```python
from build123d import *

# Parameters (mm, degrees)
SKETCH1_W           = 20.32
SKETCH1_H           = 76.2
BOSS_EXTRUDE1_DEPTH = 22.86
SKETCH2_R           = 3.175
CUT_EXTRUDE1_DEPTH  = 92.1573409
SKETCH3_W           = 20.32
SKETCH3_H           = 45.72
BOSS_EXTRUDE2_DEPTH = 50.8
SKETCH4_R           = 17.999964
CUT_EXTRUDE2_DEPTH  = 17.78
SKETCH5_R           = 2.999994
CUT_EXTRUDE3_DEPTH  = 131.260155074


with BuildPart() as part:
    # Sketch1 → Boss-Extrude1 (new, symmetric)
    with BuildSketch(Plane.XY):
        with Locations((10.16, 38.1)):
            Rectangle(SKETCH1_W, SKETCH1_H)
    extrude(amount=BOSS_EXTRUDE1_DEPTH, both=True)

    # Sketch2 → Cut-Extrude1 (cut, through all)
    with BuildSketch(Plane.XY.offset(22.86)):
        with Locations((10.16, 12.7)):
            Circle(SKETCH2_R)
        with Locations((10.16, 38.1)):
            Circle(SKETCH2_R)
        with Locations((10.16, 63.5)):
            Circle(SKETCH2_R)
    extrude(amount=-CUT_EXTRUDE1_DEPTH, mode=Mode.SUBTRACT)

    # Sketch3 → Boss-Extrude2 (add)
    with BuildSketch(Plane(origin=(0, 76.2, 0), x_dir=(1, 0, 0), z_dir=(0, 1, 0))):
        with Locations((10.16, 0)):
            Rectangle(SKETCH3_W, SKETCH3_H)
    extrude(amount=BOSS_EXTRUDE2_DEPTH)

    # Sketch4 → Cut-Extrude2 (cut)
    with BuildSketch(Plane(origin=(20.32, 0, 0), x_dir=(0, 0, -1), z_dir=(1, 0, 0))):
        with Locations((0, 96.300036)):
            Circle(SKETCH4_R)
    extrude(amount=-CUT_EXTRUDE2_DEPTH, mode=Mode.SUBTRACT)

    # Sketch5 → Cut-Extrude3 (cut, through all)
    with BuildSketch(Plane(origin=(2.54, 0, 0), x_dir=(0, 0, -1), z_dir=(1, 0, 0))):
        with Locations((0, 96.300036)):
            Circle(SKETCH5_R)
    extrude(amount=-CUT_EXTRUDE3_DEPTH, mode=Mode.SUBTRACT)


solid = part.part
```
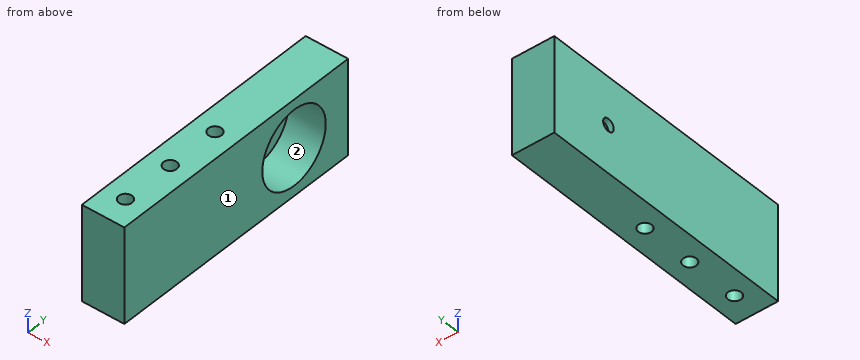
The listing builds one solid part. Answer for the finished solid, in the listing's coordinates (mm). Face numbers are marked on the shaded views. A direction names the side the tool comes from. Round coordinates to 2 decimals unless told otherwise and drop trailing zeros. Write each loop counter-clockwise with the first axis right and the second up, starting at its lowest first coordinate (ties: lowest second). Pieces come first, ordered by that corner, then holes. Notation, with made-up numbers: (14.25, 27) -> (70.25, 27) arc R14 cw to (70.25, 38) -> close; hole circle Ø10 at (79, 41). An arc over 180 degrees is marked (long way). Answer as a JSON object with one key per item and string values. Group by question number.
Q1. Section C-C (x = 10.16) is taken. Write down the section's boundary in (y, z) (3 decimals), plus the area to 3 significant figures.
Q2. Section D-D (z = -5) is taken. Write down the section's boundary in (x, y) (3 decimals), plus the area to 3 significant figures.
Q3. Section B-B (z = 0) is taken. Write down the section's boundary in (x, y) (3 decimals).
Q4. Each of these flat-tipped pins is pushed along its axis until it touches: pin 1 Ø12 at (y, z) = (71.5, -7) entering from -X; pin 2 Ø5.5 at (y, z) = (96.3, 0) entering from +X. Where does it stop, or does it pass through?
Q5. Straight lines are drawn through the part: line 1 along Y through (x, z) = (1.75, 0); line 2 along Y through (x, z) = (9.25, 0); line 3 along Y through (x, z) = (10.16, 7) (3 decimals). For each, find the intervals that lie inside material, in ascending order.
Q6. Section A-A (y = 63.5) is taken. Write down the section's boundary in (x, z) (3 decimals), plus the area to 3 significant figures.
Q7. Which of the six approach directions +Z, -Z, +X, -X, +Y, -Y give full straight-line access (tool end or side, diameter ignored) to the marked faces 1 and 2?
Check values:
{
 "1": {"outline": "(0, -22.86) -> (9.525, -22.86) -> (9.525, 22.86) -> (0, 22.86) -> close; (15.875, -22.86) -> (34.925, -22.86) -> (34.925, 22.86) -> (15.875, 22.86) -> close; (41.275, -22.86) -> (60.325, -22.86) -> (60.325, 22.86) -> (41.275, 22.86) -> close; (66.675, -22.86) -> (127, -22.86) -> (127, 22.86) -> (66.675, 22.86) -> close; hole circle Ø36 at (96.3, 0)", "area": "3,920 mm^2"},
 "2": {"outline": "(0, 0) -> (20.32, 0) -> (20.32, 79.008) -> (2.54, 79.008) -> (2.54, 113.592) -> (20.32, 113.592) -> (20.32, 127) -> (0, 127) -> close; hole circle Ø6.35 at (10.16, 12.7); hole circle Ø6.35 at (10.16, 38.1); hole circle Ø6.35 at (10.16, 63.5)", "area": "1,870 mm^2"},
 "3": {"outline": "(0, 0) -> (20.32, 0) -> (20.32, 78.3) -> (2.54, 78.3) -> (2.54, 93.3) -> (0, 93.3) -> close; (0, 99.3) -> (2.54, 99.3) -> (2.54, 114.3) -> (20.32, 114.3) -> (20.32, 127) -> (0, 127) -> close; hole circle Ø6.35 at (10.16, 12.7); hole circle Ø6.35 at (10.16, 38.1); hole circle Ø6.35 at (10.16, 63.5)"},
 "4": {"pin 1": "x = 0", "pin 2": "through"},
 "5": {"line 1": "0 to 93.3, 99.3 to 127", "line 2": "0 to 9.66, 15.74 to 35.06, 41.14 to 60.46, 66.54 to 78.3, 114.3 to 127", "line 3": "0 to 9.525, 15.875 to 34.925, 41.275 to 60.325, 66.675 to 79.717, 112.883 to 127"},
 "6": {"outline": "(0, -22.86) -> (6.985, -22.86) -> (6.985, 22.86) -> (0, 22.86) -> close; (13.335, -22.86) -> (20.32, -22.86) -> (20.32, 22.86) -> (13.335, 22.86) -> close", "area": "639 mm^2"},
 "7": {"face 1": "+Z, -Z, +X, +Y, -Y", "face 2": "+X"}
}
